```python
from build123d import *

# Parameters (mm, degrees)
F0_R     = 9.5
F0_R_2   = 8
F1_DEPTH = 150
F3_W     = 20
F3_H     = 30
F4_DEPTH = 30
F5_R     = 10
F9_R     = 2


with BuildPart() as f1:
    # F0 (on Top) → F1 (new body)
    with BuildSketch(Plane.XY):
        Circle(F0_R)
        Circle(F0_R_2, mode=Mode.SUBTRACT)
    extrude(amount=F1_DEPTH)


with BuildPart() as f4:
    # F3 (on Top) → F4 (new body)
    with BuildSketch(Plane.XY):
        Rectangle(F3_W, F3_H)
    extrude(amount=F4_DEPTH)

    # F5
    f5_edges = [f4.edges().sort_by_distance(p)[0] for p in [
        (0, 15, 30),
    ]]
    fillet(f5_edges, radius=F5_R)

    # F8: sweep along a path in F6
    with BuildLine(Plane.YZ) as f8_path:
        Line((15, 0), (15, 20))
        ThreePointArc((15, 20), (12.0710678119, 27.0710678119), (5, 30))
        Line((5, 30), (-15.0585370138, 30))
    # F7 (on face) → F8 (sweep, cut)
    with BuildSketch(Plane(origin=(0, 0, 0), x_dir=(1, 0, 0), z_dir=(0, 0, -1))):
        with BuildLine():
            Line((-2.75, -15), (2.75, -15))
            ThreePointArc((2.75, -15), (0, -12.25), (-2.75, -15))
        make_face()
    sweep(path=f8_path.line, mode=Mode.SUBTRACT)

    # F9
    f9_edges = [f4.edges().sort_by_distance(p)[0] for p in [
        (0, 5, 27.25),
        (-2.75, -5, 30),
        (0, -15, 27.25),
        (2.75, -5, 30),
        (2.75, 12.071068, 27.071068),
        (0, 12.25, 20),
        (-2.75, 12.071068, 27.071068),
        (2.75, 15, 10),
        (0, 12.25, 0),
        (-2.75, 15, 10),
        (-10, 12.071068, 27.071068),
        (10, 12.071068, 27.071068),
        (10, 15, 10),
        (10, 0, 0),
        (10, -5, 30),
        (10, -15, 15),
        (-10, 15, 10),
        (-10, 0, 0),
        (-10, -5, 30),
        (-10, -15, 15),
        (0, -15, 0),
        (-6.375, 15, 0),
        (6.375, 15, 0),
        (6.375, -15, 30),
        (-6.375, -15, 30),
    ]]
    fillet(f9_edges, radius=F9_R)


solid = f4.part
```
For this review, take the finished solid that the model builds, in its own axes (mm). A direction names the side the tool comes from. Coordinates: 2 decimals unless noted, no trailing zeros. Order: outer loops, then holes, each group sorted by start corner. A loop starts at its lowest first (then second) coordinate and runs counter-clockwise, first axis right, second up. Notation, with made-up numbers: (63.25, -33) -> (75.25, -33) arc R9 cw to (75.25, -20) -> close; hole circle Ø10 at (38.5, 42). An arc over 180 degrees is marked (long way). Use CSV: the item, a comma, the result in double quotes. Start each with the question number.
Item 1: For faces 1 (the face through (-3.246, -4.126, 29.694)), 2 (the face through (6.18, 14.4, 0.57)), 3 (the face through (3.22, 14.68, 11.13)), list the 3-axis set-ups (+Z, -Z, +X, -X, +Y, -Y) from which the entire face can be reached by the end or side of a thin tool; tool diameter is ignored.
Item 2: Wall thickness on probe 1 along X at (y, z) = (10, 26); probe 2 along X at (y, z) = (10, 27); probe 3 along Y at (x, z) = (1.5, 25.5): over which ranges is each line inside the solid? List them lowest first.
Item 3: Insertion check: pin 1 (1 mm diameter, centred on x = 0, y = 5.5, fed in from +Z). The pin has a flat end and moves straight along its axis. Give the tip position at first contact, or say it passes through.
Item 4: We need section B-B, the plane z = 12. Give the boundary of the cut face in (x, y).
Item 5: Draft analysis for pull direction X (two halves, no side actions). For faces 4 (the face through (-6.13, 14.43, 0.6)), 5 (the face through (-0.04, 12.25, 11.13)), 6 (the face through (-9.43, -4.13, 29.4)), state which applies: pulls with the +X half, pulls with the -X half, needs draft (parallel to the pull), parting line crosses it, or undercut.
Item 6: We need section A-A, the plane x = -6.75. Give the boundary of the cut face in (y, z), then the cut area to 3 significant figures.
Item 7: We need section C-C, the plane y = -1. Give the boundary of the cut face in (x, z).
Derived:
1,face 1,"+Z, +Y, -Y"
1,face 2,"-Z, +X, -X, +Y"
1,face 3,"+Z, -Z, +Y"
2,probe 1,"x = -10 to -1.66, 1.66 to 10"
2,probe 2,"x = -9.91 to -2.37, 2.37 to 9.91"
2,probe 3,"y = -15 to 10.38"
3,pin 1,"stops at z = 27.28"
4,outline,"(-10, -13) arc R2 ccw to (-8, -15) -> (8, -15) arc R2 ccw to (10, -13) -> (10, 13) arc R2 ccw to (8, 15) -> (4.31, 15) arc R2 ccw to (2.49, 13.84) arc R2.75 cw to (-2.49, 13.84) arc R2 ccw to (-4.31, 15) -> (-8, 15) arc R2 ccw to (-10, 13) -> close"
5,face 4,"needs draft"
5,face 5,"undercut"
5,face 6,"pulls with the -X half"
6,outline,"(-15, 2) arc R2 ccw to (-13, 0) -> (13, 0) arc R2 ccw to (15, 2) -> (15, 20) arc R10 ccw to (5, 30) -> (-13, 30) arc R2 ccw to (-15, 28) -> close"
6,area,"876 mm^2"
7,outline,"(-10, 2) arc R2 ccw to (-8, 0) -> (8, 0) arc R2 ccw to (10, 2) -> (10, 28) arc R2 ccw to (8, 30) -> (4.31, 30) arc R2 ccw to (2.49, 28.84) arc R2.75 cw to (-2.49, 28.84) arc R2 ccw to (-4.31, 30) -> (-8, 30) arc R2 ccw to (-10, 28) -> close"
